```python
from build123d import *

# Parameters (mm, degrees)
EXTRUDE_1_DEPTH             = 15
CUT_EXTRUDE_1_DEPTH         = 9
FILLET_1_R                  = 2
CUT_EXTRUDE_2_REACH         = 33.337
SKETCH_4_R                  = 1.5000000000000007
CUT_EXTRUDE_3_DEPTH         = 45.068129073061414
SKETCH_6_W                  = 1.5
SKETCH_6_H                  = 6
CUT_EXTRUDE_5_DEPTH         = 39.8587184554509
CUT_EXTRUDE_4_DEPTH         = 6
SKETCH_7_W                  = 22.5
SKETCH_7_H                  = 5
EXTRUDE_2_DEPTH             = 0.5
FILLET_2_R                  = 0.5
HOLE_WIZARD_2_2_2_2_1_D     = 2.2
HOLE_WIZARD_2_2_2_2_1_DEPTH = 2
MIRROR_2_COPY_1_DEPTH       = 6
SKETCH_10_W                 = 26.000000000000004
SKETCH_10_H                 = 2.9999999999999964
CUT_EXTRUDE_6_DEPTH         = 36.59494346111538
EXTRUDE_3_DEPTH             = 0.75
MIRROR_4_COPY_1_DEPTH       = 0.75


with BuildPart() as part:
    # ｽｹｯﾁ1 → ﾎﾞｽ - 押し出し1 (new, symmetric)
    with BuildSketch(Plane(origin=(0, 0, 0), x_dir=(0, 0, -1), z_dir=(1, 0, 0))):
        with BuildLine():
            Line((8.999999999999996, 31.000000000000004), (0.2508278236462402, 31))
            ThreePointArc((0.2508278236462402, 31), (-6.627408015078736, 17.74430242011084), (-9, 3))
            Line((-9, 3), (-9, -3))
            Line((-9, -3), (9, -2.999999999999999))
            Line((9, -2.999999999999999), (8.999999999999996, 31.000000000000004))
        make_face()
    extrude(amount=EXTRUDE_1_DEPTH, both=True)

    # ｽｹｯﾁ2 → ｶｯﾄ - 押し出し1 (cut)
    with BuildSketch(Plane(origin=(0, 9.2e-16, -9), x_dir=(-1, 0, 0), z_dir=(0, 1e-16, -1))):
        Polygon((-13, 31.000000000000004), (13, 31.000000000000004), (13.000000000000002, 5), (-12.999999999999996, 5), align=None)
    extrude(amount=-CUT_EXTRUDE_1_DEPTH, mode=Mode.SUBTRACT)

    # ﾌｨﾚｯﾄ1
    fillet_1_edges = [part.edges().sort_by_distance(p)[0] for p in [
        (-14, 31.000000000000004, -8.999999999999996),
    ]]
    fillet(fillet_1_edges, radius=FILLET_1_R)
    fillet_1_2_edges = [part.edges().sort_by_distance(p)[0] for p in [
        (14, 31.000000000000004, -8.999999999999996),
    ]]
    fillet(fillet_1_2_edges, radius=FILLET_1_R)
    fillet_1_3_edges = [part.edges().sort_by_distance(p)[0] for p in [
        (-14, 31, -0.2508278236462367),
    ]]
    fillet(fillet_1_3_edges, radius=FILLET_1_R)

    # ｽｹｯﾁ3 → ｶｯﾄ - 押し出し2 (cut, up to next)
    with BuildSketch(Plane(origin=(0, 5, 5.1e-16), x_dir=(1, 0, 0), z_dir=(0, 1, 1e-16)), mode=Mode.PRIVATE) as cut_extrude_2_sk1:
        Polygon((-8.749999999999998, 9), (8.750000000000002, 9), (8.750000000000004, 5.999999999999999), (-8.749999999999998, 5.999999999999999), align=None)
    cut_extrude_2_tool1 = extrude(cut_extrude_2_sk1.sketch, amount=-CUT_EXTRUDE_2_REACH, mode=Mode.PRIVATE) & part.part
    add(cut_extrude_2_tool1.solids().sort_by_distance((0, 5, -7.5))[0], mode=Mode.SUBTRACT)

    # ｽｹｯﾁ4 → ｶｯﾄ - 押し出し3 (cut, through all)
    with BuildSketch(Plane(origin=(15, 0, 0), x_dir=(0, 0, -1), z_dir=(1, 0, 0))):
        Circle(SKETCH_4_R)
    extrude(amount=-CUT_EXTRUDE_3_DEPTH, mode=Mode.SUBTRACT)

    # ｽｹｯﾁ6 → ｶｯﾄ - 押し出し5 (cut, through all)
    with BuildSketch(Plane.XY.offset(9)):
        Polygon((-15, 3), (-13.5, 3), (-13.499999999999998, -3), (-15, -3), align=None)
        with Locations((14.250000000000002, 0)):
            Rectangle(SKETCH_6_W, SKETCH_6_H)
    extrude(amount=-CUT_EXTRUDE_5_DEPTH, mode=Mode.SUBTRACT)

    # ｽｹｯﾁ5 → ｶｯﾄ - 押し出し4 (cut)
    with BuildSketch(Plane.XZ.offset(2.9999999999999996)):
        Polygon((13.5, -3), (10, -4.500000000000001), (10, -7), (13.5, -7.9), align=None)
    cut_extrude_4 = extrude(amount=-CUT_EXTRUDE_4_DEPTH, mode=Mode.SUBTRACT)

    # ﾐﾗｰ1: ｶｯﾄ - 押し出し4 across plane
    add(cut_extrude_4.mirror(Plane.XY), mode=Mode.SUBTRACT)

    # ｽｹｯﾁ7 → ﾎﾞｽ - 押し出し2 (add)
    with BuildSketch(Plane.XZ.offset(2.9999999999999996)):
        Rectangle(SKETCH_7_W, SKETCH_7_H)
    extrude(amount=EXTRUDE_2_DEPTH)

    # ﾌｨﾚｯﾄ2
    fillet_2_edges = [part.edges().sort_by_distance(p)[0] for p in [
        (11.250000000000004, -3.2499999999999996, -2.5000000000000004),
        (11.250000000000004, -3.2499999999999996, 2.4999999999999996),
        (-11.249999999999996, -3.2499999999999996, 2.4999999999999996),
        (-11.249999999999996, -3.2499999999999996, -2.5000000000000004),
        (11.250000000000004, -3.4999999999999996, -6.1e-16),
        (3.55e-15, -3.4999999999999996, 2.4999999999999996),
        (-11.249999999999996, -3.4999999999999996, -6.1e-16),
        (3.55e-15, -3.4999999999999996, -2.5000000000000004),
    ]]
    fillet(fillet_2_edges, radius=FILLET_2_R - 0.0001)  # a hair under: the kernel refuses the full size

    # Ø2.2 (2.2) 直径の穴1
    with Locations(Plane(origin=(15, 0, 0), x_dir=(0, 0, -1), z_dir=(1, 0, 0))):
        with Locations((2.5, 28.5), (2.5, 7.5)):
            hole_wizard_2_2_2_2_1 = Hole(HOLE_WIZARD_2_2_2_2_1_D / 2, depth=HOLE_WIZARD_2_2_2_2_1_DEPTH)

    # ﾐﾗｰ2: ｶｯﾄ - 押し出し4, Ø2.2 (2.2) 直径の穴1 across plane
    add(cut_extrude_4.mirror(Plane(origin=(0, 0, 0), x_dir=(0, 0, 1), z_dir=(1, 0, 0))), mode=Mode.SUBTRACT)
    add(hole_wizard_2_2_2_2_1.mirror(Plane(origin=(0, 0, 0), x_dir=(0, 0, 1), z_dir=(1, 0, 0))), mode=Mode.SUBTRACT)

    # ﾐﾗｰ2 copy 1 sketch → ﾐﾗｰ2 copy 1 (cut)
    with BuildSketch(Plane(origin=(0, -2.9999999999999996, 1.4e-16), x_dir=(-1, 0, 0), z_dir=(0, -1, 5e-17))):
        Polygon((13.5, -3), (10, -4.500000000000001), (10, -7), (13.5, -7.9), align=None)
    extrude(amount=-MIRROR_2_COPY_1_DEPTH, mode=Mode.SUBTRACT)

    # ｽｹｯﾁ10 → ｶｯﾄ - 押し出し6 (cut, through all)
    with BuildSketch(Plane(origin=(0, 0, 0), x_dir=(-1, 0, 0), z_dir=(0, 1.3e-16, -1))):
        with Locations((0, 31.5)):
            Rectangle(SKETCH_10_W, SKETCH_10_H)
    extrude(amount=-CUT_EXTRUDE_6_DEPTH, mode=Mode.SUBTRACT)

    # ｽｹｯﾁ12 → ﾎﾞｽ - 押し出し3 (add, symmetric)
    with BuildSketch(Plane(origin=(0, 0, 0), x_dir=(-1, 0, 0), z_dir=(0, -1, -2e-17))):
        Polygon((13.5, -7.9), (9.999999999999998, -7), (10, -6.500000000000001), (13.5, -7.4), align=None)
        Polygon((10, -4.500000000000001), (10, -5), (13.499999999999998, -3.4999999999999982), (13.5, -2.9999999999999996), align=None)
    extrude_3 = extrude(amount=EXTRUDE_3_DEPTH, both=True)

    # ﾐﾗｰ3: ﾎﾞｽ - 押し出し3 across plane
    add(extrude_3.mirror(Plane.XY))

    # ﾐﾗｰ4: ﾎﾞｽ - 押し出し3 across plane
    add(extrude_3.mirror(Plane(origin=(0, 0, 0), x_dir=(0, 0, 1), z_dir=(1, 0, 0))))

    # ﾐﾗｰ4 copy 1 sketch → ﾐﾗｰ4 copy 1 (add, symmetric)
    with BuildSketch(Plane.XZ):
        Polygon((13.5, -7.9), (9.999999999999998, -7), (10, -6.500000000000001), (13.5, -7.4), align=None)
        Polygon((10, -4.500000000000001), (10, -5), (13.499999999999998, -3.4999999999999982), (13.5, -2.9999999999999996), align=None)
    extrude(amount=MIRROR_4_COPY_1_DEPTH, both=True)


solid = part.part
```
For this review, take the finished solid that the model builds, in its own axes (mm). A direction names the side the tool comes from. Round coordinates to 2 decimals unless told otherwise and drop trailing zeros. Write each loop counter-clockwise with the first axis right and the second up, starting at its lowest first coordinate (ties: lowest second). Pieces come first, ordered by that corner, then holes. Notation, with made-up numbers: (58.25, 30) -> (81.25, 30) arc R10 ccw to (81.25, 49) -> close; hole circle Ø5 at (-30.75, -21). An arc over 180 degrees is marked (long way). One line per question, with ' | ' between items. Start each with the question number.
1) For pin 1 Ø1.5 at (x, z) = (-12, -2.5) entering from -Y; pin 2 Ø0.7 at (x, z) = (11.5, -7) entering from +Y; pin 3 Ø1.8 at (y, z) = (1.5, 0.5) entering from +X, all flat-tipped, find the tip position at first contact; note any pin that passes through.
2) Mouldability with a two-part tool opening along Y and no side actions: class faces 1 (the cylindrical face through (0.189, -1.464, 0.325)), 2 (the cylindrical face through (13.99, 7.83, -1.45)), 3 (the flat face through (-11.74, -0.75, -3.92)), 4 (the flat face through (-11.726, 0.01, 6.944)) as +Y half, -Y half, draft (parallel to the pull), parting line (faces both ways), or undercut.
3) Machinability: for faces 5 (the flat face through (11.726, -1.891, 7.444)), 6 (the flat face through (13.5, 0, 2)), 7 (the flat face through (-13.5, 0, 8)), 8 (the flat face through (-11.76, -0.75, -7.14)), 9 (the flat face through (0, 5, -4)), which of the approach directions +Z, -Z, +X, -X, +Y, -Y give a long, thin tool a straight path to every point of the face, cutting with its end or side? Answer none if there is none.
4) Add section A-A (y = 0). Write out the cut boundary in (x, z), and give its area (3 significant figures).
5) Add section C-C (y = 28.5). Write out the cut boundary in (x, z), and give its area (3 significant figures).
6) Wall thickness on line 1 along Y through (x, z) = (13.9, -2.5); line 2 along X through (y, z) = (10, -7.25); line 3 along Y through (x, z) = (11, -4.5): over which ranges is each line inside the solid? List them lowest first.
Reported:
1) pin 1: stops at y = -3 | pin 2: stops at y = 5 | pin 3: stops at x = 13.5
2) face 1: undercut | face 2: undercut | face 3: -Y half | face 4: draft
3) face 5: +X, -Y | face 6: +Z, -Z, +X, -Y | face 7: +Z, -Z, -X, -Y | face 8: -X, -Y | face 9: -Z, +Y
4) outline: (-13.5, -9) -> (-8.75, -9) -> (-8.75, -6) -> (8.75, -6) -> (8.75, -9) -> (13.5, -9) -> (13.5, -7.4) -> (10, -6.5) -> (10, -5) -> (13.5, -3.5) -> (13.5, -1.5) -> (-13.5, -1.5) -> (-13.5, -3.5) -> (-10, -5) -> (-10, -6.5) -> (-13.5, -7.4) -> close; (-13.5, 1.5) -> (13.5, 1.5) -> (13.5, 3.5) -> (10, 5) -> (10, 6.5) -> (13.5, 7.4) -> (13.5, 9) -> (-13.5, 9) -> (-13.5, 7.4) -> (-10, 6.5) -> (-10, 5) -> (-13.5, 3.5) -> close | area: 315 mm²
5) outline: (-15, -9) -> (-13, -9) -> (-13, -3.6) -> (-15, -3.6) -> close; (-15, -1.4) -> (-13, -1.4) -> (-13, 0) -> (13, 0) -> (13, -1.4) -> (15, -1.4) -> (15, 1.48) -> (-15, 1.48) -> close; (13, -9) -> (15, -9) -> (15, -3.6) -> (13, -3.6) -> close | area: 71.6 mm²
6) line 1: y = 3 to 6.4, 8.6 to 27.4, 29.6 to 31 | line 2: x = -15 to -13, 13 to 15 | line 3: y = -0.75 to 0.75, 3 to 5
